CAD build for the part. Positions are in the model's coordinates, mm. A direction names the side the tool comes from. Round coordinates to 2 decimals unless told otherwise and drop trailing zeros. Loops run counter-clockwise (first coordinate to the right, second up) from the corner with the lowest first, then second, coordinate; pieces in that order, holes last.
from build123d import *

# Parameters (mm, degrees)
SKETCH1_W           = 65
SKETCH1_H           = 32
BOSS_EXTRUDE1_DEPTH = 2
SKETCH3_W           = 25
SKETCH3_H           = 2
BOSS_EXTRUDE2_DEPTH = 14
FILLET1_R           = 15
SKETCH4_R           = 2
CUT_EXTRUDE2_DEPTH  = 33
SKETCH2_R           = 8
BOSS_EXTRUDE3_DEPTH = 8


with BuildPart() as part:
    # Sketch1 → Boss-Extrude1 (new body)
    with BuildSketch(Plane.XY):
        Rectangle(SKETCH1_W, SKETCH1_H)
    extrude(amount=BOSS_EXTRUDE1_DEPTH)

    # Sketch3 → Boss-Extrude2 (add)
    with BuildSketch(Plane(origin=(0, 0, 0), x_dir=(-1, 0, 0), z_dir=(0, 0, -1))):
        with Locations((0, 15)):
            Rectangle(SKETCH3_W, SKETCH3_H)
    extrude(amount=BOSS_EXTRUDE2_DEPTH)

    # Fillet1
    fillet1_edges = [part.edges().sort_by_distance(p)[0] for p in [
        (32.5, -16, 1),
        (-32.5, -16, 1),
    ]]
    fillet(fillet1_edges, radius=FILLET1_R)

    # Sketch4 → Cut-Extrude2 (cut, through all)
    with BuildSketch(Plane(origin=(0, 16, 0), x_dir=(1, 0, 0), z_dir=(0, 1, 0))):
        with Locations((0, 7)):
            Circle(SKETCH4_R)
    extrude(amount=-CUT_EXTRUDE2_DEPTH, mode=Mode.SUBTRACT)

    # Sketch2 → Boss-Extrude3 (add)
    with BuildSketch(Plane.XY.offset(2)):
        with Locations((-12.5, -1)):
            Circle(SKETCH2_R)
        with Locations((12.5, -1)):
            Circle(SKETCH2_R)
    extrude(amount=BOSS_EXTRUDE3_DEPTH)


solid = part.part
Item 1: 3-axis set-ups, long thin cutter, end or side, ignore diameter. For faces 1 (the flat face through (12.5, 15, -7)), 2 (the flat face through (-12.5, 15, -7)), 3 (the flat face through (3, 14, -7)), 4 (the flat face through (0, 0, 2)): which of +Z, -Z, +X, -X, +Y, -Y reach the whole face in a straight line?
Verdict:
face 1: -Z, +X, +Y, -Y
face 2: -Z, -X, +Y, -Y
face 3: -Z, +X, -X, -Y
face 4: +Z
Item 2: Cut at D-D (x = 15). List the corners of the cut face in (y, z), plus the area to 3 significant figures.
Verdict:
outline: (-16, 0) - (16, 0) - (16, 2) - (6.6, 2) - (6.6, 10) - (-8.6, 10) - (-8.6, 2) - (-16, 2) - close
area: 186 mm2
Item 3: Flat gauge pins, fed straight in: P1, Ø4, axis at x = 2, z = -4, coming from the -Y side; P2, Ø8, axis at x = 22.5, z = -5, coming from the -Y side; P3, Ø6, axis at x = 5, y = -12, coming from the +Z side; P4, Ø1.6, axis at y = 14.5, z = -10, coming from the -X side. Where does each tip first touch, or does it go through?
Verdict:
P1: stops at y = 14
P2: passes through
P3: stops at z = 2
P4: stops at x = -12.5
Item 4: Wall check: L1, parallel to Z at x = 0, y = 14.5; L2, parallel to X at y = 15.4, z = -7; L3, parallel to X at y = -3.5, z = 4. Give the ranges that are in metal, low to high.
Verdict:
L1: z = -14 to -9, -5 to 2
L2: x = -12.5 to -2, 2 to 12.5
L3: x = -20.1 to -4.9, 4.9 to 20.1
Item 5: Cut at A-A (x = 0). List the corners of the cut face in (y, z), plus the area to 3 significant figures.
Verdict:
outline: (-16, 0) - (14, 0) - (14, -5) - (16, -5) - (16, 2) - (-16, 2) - close; (14, -14) - (16, -14) - (16, -9) - (14, -9) - close
area: 84.0 mm2
Item 6: Cut at C-C (y = -3). List the corners of the cut face in (x, z), plus the area to 3 significant figures.
Verdict:
outline: (-32.37, 0) - (32.37, 0) - (32.37, 2) - (20.25, 2) - (20.25, 10) - (4.75, 10) - (4.75, 2) - (-4.75, 2) - (-4.75, 10) - (-20.25, 10) - (-20.25, 2) - (-32.37, 2) - close
area: 377 mm2
Item 7: Mould opens along X. For faces 5 (the flat face through (0, 16, -4)), 6 (the cylindrical face through (27.99, -11.72, 1.01)), 7 (the flat face through (-32.5, 7, 1)), 8 (the cylindrical face through (10.77, -8.81, 5.94)) say: released by +X, released by -X, zero draft, split by the parting line, or undercut.
Verdict:
face 5: zero draft
face 6: released by +X
face 7: released by -X
face 8: undercut
Item 8: Cut at B-B (z = 8). List the corners of the cut face in (x, y).
Verdict:
outline: circle Ø16 at (-12.5, -1); circle Ø16 at (12.5, -1)
